Part model, mm, in its own coordinate system. Give positions to 0.01 mm unless a question says otherwise; leave off trailing zeros. Use a Markdown table: item, result. Add a question column.
from build123d import *

# Parameters (mm, degrees)
CROQUIS1_W              = 214
CROQUIS1_H              = 314
CROQUIS1_R              = 1.55
SALIENTE_EXTRUIR1_DEPTH = 4.7


with BuildPart() as part:
    # Croquis1 → Saliente-Extruir1 (new body)
    with BuildSketch(Plane(origin=(0, 0, 0), x_dir=(1, 0, 0), z_dir=(0, 1, 0))):
        with Locations((107, 157)):
            Rectangle(CROQUIS1_W, CROQUIS1_H)
        with Locations(Location((2.5, 311.5, 0), (0, 0, 270))):
            Circle(CROQUIS1_R, mode=Mode.SUBTRACT)
        with Locations(Location((211.5, 311.5, 0), (0, 0, 90))):
            Circle(CROQUIS1_R, mode=Mode.SUBTRACT)
        with Locations(Location((2.5, 2.5, 0), (0, 0, 90))):
            Circle(CROQUIS1_R, mode=Mode.SUBTRACT)
        with Locations(Location((211.5, 2.5, 0), (0, 0, 270))):
            Circle(CROQUIS1_R, mode=Mode.SUBTRACT)
        with Locations(Location((5.5, 157, 0), (0, 0, 270))):
            Circle(CROQUIS1_R, mode=Mode.SUBTRACT)
        with Locations(Location((208.5, 157, 0), (0, 0, 90))):
            Circle(CROQUIS1_R, mode=Mode.SUBTRACT)
    extrude(amount=SALIENTE_EXTRUIR1_DEPTH)


solid = part.part
1. Pin check, flat tip, straight feed: P1, Ø4, axis at x = 2.5, z = -2.5, coming from the -Y side. Stop position of the tip, or through.
2. Mould opens along Y. For faces 1 (the face through (106, 4.7, -159)), 2 (the face through (106, 0, -159)) say: released by +Y, released by -Y, zero draft, split by the parting line, or undercut.
3. Drill centre lines: probe 1 along X at (y, z) = (3.7, -311.5); probe 2 along X at (y, z) = (2.1, -157); probe 3 along Z at (x, y) = (211.5, 1.3). Where is each one in solid material? Low to high. Write a range as [from, to].
Responses:
| question | item | result |
|---|---|---|
| 1 | P1 | stops at y = 0 |
| 2 | face 1 | released by +Y |
| 2 | face 2 | released by -Y |
| 3 | probe 1 | x = [0, 0.95], [4.05, 209.95], [213.05, 214] |
| 3 | probe 2 | x = [0, 3.95], [7.05, 206.95], [210.05, 214] |
| 3 | probe 3 | z = [-314, -313.05], [-309.95, -4.05], [-0.95, 0] |
